Geometry: final body of the model. Coordinates: model frame, mm. A direction names the side the tool comes from. Give positions to 0.01 mm unless a question says otherwise; leave off trailing zeros. Write each loop counter-clockwise with the first axis right and the second up, starting at its lowest first coordinate (ties: lowest second). Pieces come first, ordered by that corner, then holes. Notation, with made-up numbers: (25.25, 44) -> (50.25, 44) arc R33 cw to (50.25, 79) -> close; hole circle Ø2 at (8, 14). An arc over 180 degrees is marked (long way). Answer as a JSON object with one key per item and string values.
from build123d import *

# Parameters (mm, degrees)
F1_DEPTH = 10
F0_W     = 24.7
F0_H     = 20
F2_DEPTH = 5
F5_DEPTH = 24.7
F6_DEPTH = 40
F9_DEPTH = 24.7


with BuildPart() as f1:
    # F0 (on Top) → F1 (new body)
    with BuildSketch(Plane.XY):
        Polygon((-20, 25), (-20, 15), (-20, -5), (-20, -15), (20, -15), (20, -5), (20, 15), (20, 25), align=None)
    extrude(amount=F1_DEPTH)

    # F0 (on Top) → F2 (join)
    with BuildSketch(Plane.XY):
        with Locations((-32.35, 5)):
            Rectangle(F0_W, F0_H)
        Polygon((-20, 25), (-20, 15), (-20, -5), (-20, -15), (20, -15), (20, -5), (20, 15), (20, 25), align=None)
        with Locations((32.35, 5)):
            Rectangle(F0_W, F0_H)
    extrude(amount=F2_DEPTH)

    # F4 (on offset) → F5 (join)
    with BuildSketch(Plane.YZ.offset(20)):
        Polygon((-5, 5), (15, 5), (8.7127050693, 10), (1.2872949307, 10), align=None)
        Polygon((1.2872949307, 10), (8.7127050693, 10), (5, 12.9525456578), align=None)
    extrude(amount=F5_DEPTH)

    # F4 (on offset) → F6 (join)
    with BuildSketch(Plane.YZ.offset(20)):
        Polygon((5, 12.9525456578), (8.7127050693, 10), (25, 10), (5, 26.0377600789), (-15, 10), (1.2872949307, 10), align=None)
        Polygon((1.2872949307, 10), (8.7127050693, 10), (5, 12.9525456578), align=None)
    extrude(amount=-F6_DEPTH)

    # F8 (on offset) → F9 (join)
    with BuildSketch(Plane(origin=(-20, 0, 0), x_dir=(0, -1, 0), z_dir=(-1, 0, 0))):
        Polygon((-15, 5), (5, 5), (-5, 13.4582445025), align=None)
    extrude(amount=F9_DEPTH)


solid = f1.part
Q1. Cut plane D-D (x = 17). Return the cut outline in (y, z).
Values:
{"outline": "(-15, 0) -> (25, 0) -> (25, 10) -> (5, 26.04) -> (-15, 10) -> close"}
Q2. Cut plane A-A (x = 33). Return the cut outline in (y, z).
Values:
{"outline": "(-5, 0) -> (15, 0) -> (15, 5) -> (5, 12.95) -> (-5, 5) -> close"}
Q3. Material intervals for L1, parallel to X at y = 23, z = 2; L2, parallel to Y at x = -37.5, z = 9.5; L3, parallel to Y at x = -34, z = 13.25, sorted ascending. Write a range as from..to.
Values:
{"L1": "-20..20", "L2": "0.32..9.68", "L3": "4.75..5.25"}
Q4. Set-up query: faces 1 (the flat face through (20, 4.7, 13.2)), 2 (the flat face through (-20, 9.2, 10.3)), 3 (the flat face through (32, -5, 2)), 4 (the flat face through (-33, -5, 2)). Return all of +Z, -Z, +X, -X, +Y, -Y with unobstructed straight access to the full face (end or side cutting, diameter ignored); none if empty.
Values:
{"face 1": "+Z, +X", "face 2": "+Z, -X", "face 3": "+Z, -Z, +X, -Y", "face 4": "+Z, -Z, -X, -Y"}
Q5. Cut plane B-B (y = 11.5). Return the cut outline in (x, z).
Values:
{"outline": "(-44.7, 0) -> (44.7, 0) -> (44.7, 7.78) -> (20, 7.78) -> (20, 20.83) -> (-20, 20.83) -> (-20, 7.96) -> (-44.7, 7.96) -> close"}
Q6. Cut plane C-C (z = 24). Return the cut outline in (x, y).
Values:
{"outline": "(-20, 2.46) -> (20, 2.46) -> (20, 7.54) -> (-20, 7.54) -> close"}
Q7. First-contact query: P1, Ø12, axis at x = 20, z = 22, coming from the -Y side; P2, Ø8, axis at x = -33, z = 4.5, coming from the +Y side; P3, Ø1.5, axis at x = -2, y = 18, coming from the +Z side. Flat tips, straight axial feed; report the tip coordinate or a pass-through.
Values:
{"P1": "y = -7.52", "P2": "y = 15", "P3": "z = 16.21"}
